Autodesk Inventor part; units mm, degrees
ref_plane "YZ Plane" through (0, 0, 0) normal (1, 0, 0) x (0, 1, 0)
ref_plane "XZ Plane" through (0, 0, 0) normal (0, 1, 0) x (-1, 0, 0)
ref_plane "XY Plane" through (0, 0, 0) normal (0, 0, 1) x (1, 0, 0)
sketch "Sketch1" plane through (0, 0, 0) normal (0, 0, 1) x (1, 0, 0)
  line L0 (0, 0) -> (25.4, 0)
  line L1 (25.4, 0) -> (25.4, 50.8)
  line L2 (25.4, 50.8) -> (0, 50.8)
  line L3 (0, 50.8) -> (0, 0)
  line L4 (23.8125, 1.5875) -> (1.5875, 1.5875)
  line L5 (1.5875, 1.5875) -> (1.5875, 49.2125)
  line L6 (1.5875, 49.2125) -> (23.8125, 49.2125)
  line L7 (23.8125, 49.2125) -> (23.8125, 1.5875)
  dimension "d0" = 25.4
  dimension "d1" = 50.8
  dimension "d2" = 1.5875
extrude "Extrusion1" add sketch "Sketch1" along normal blind 584.2
sketch "Sketch2" plane through (0, 50.8, 0) normal (0, 1, 0) x (1, 0, 0)
  line L0 (23.8125, 0) -> (1.5875, 0) construction
  line L1 (12.7, 0) -> (12.7, -12.7) construction
  line L2 (25.4, -584.2) -> (0, -584.2) construction
  line L3 (12.7, -584.2) -> (12.7, -571.5) construction
  circle A0 centre (12.7, -571.5) radius 2.5797
  circle A1 centre (12.7, -12.7) radius 2.5797
  point P0 (0, 0)
  dimension "d5" = 12.7
  dimension "d6" = 12.7
  dimension "d7" = 5.1594
extrude "Extrusion2" cut sketch "Sketch2" against normal blind 711.2
sketch "Sketch3" plane through (0, 50.8, 0) normal (0, 1, 0) x (1, 0, 0)
  circle A0 centre (12.7, -12.7) radius 2.5797 construction
  line L0 (12.7, -12.7) -> (12.7, -38.1) construction
  circle A1 centre (12.7, -38.1) radius 2.5797
  circle A2 centre (12.7, -571.5) radius 2.5797 construction
  line L1 (12.7, -571.5) -> (12.7, -546.1) construction
  circle A3 centre (12.7, -546.1) radius 2.5797
  point P0 (0, 0)
  dimension "d10" = 25.4
  dimension "d13" = 25.4
extrude "Extrusion4" cut sketch "Sketch3" against normal blind 68.2625
sketch "Sketch4" plane through (25.4, 0, 0) normal (1, 0, 0) x (0, 0, -1)
  line L0 (0, 0) -> (-584.2, 0) construction
  line L1 (0, 0) -> (-284.1625, 0) construction
  line L2 (-284.1625, 0) -> (-334.9625, 0) construction
  line L3 (-334.9625, 0) -> (-334.9625, 12.7) construction
  line L4 (-334.9625, 12.7) -> (-309.5625, 12.7) construction
  line L5 (-309.5625, 12.7) -> (-309.5625, 38.1) construction
  line L6 (-309.5625, 12.7) -> (-284.1625, 12.7) construction
  circle A0 centre (-284.1625, 12.7) radius 2.5797
  circle A1 centre (-334.9625, 12.7) radius 2.5797
  circle A2 centre (-309.5625, 38.1) radius 2.5797
  dimension "d16" = 284.1625
  dimension "d17" = 50.8
  dimension "d18" = 12.7
  dimension "d19" = 25.4
  dimension "d20" = 25.4
  dimension "d21" = 5.1594
  dimension "d22" = 5.1594
extrude "Extrusion5" cut sketch "Sketch4" against normal blind 25.4
sketch "Sketch5" plane through (0, 50.8, 0) normal (0, 1, 0) x (1, 0, 0)
  circle A0 centre (12.7, -38.1) radius 2.5797 construction
  line L0 (12.7, -38.1) -> (12.7, -63.5) construction
  circle A1 centre (12.7, -546.1) radius 2.5797 construction
  line L1 (12.7, -546.1) -> (12.7, -520.7) construction
  circle A2 centre (12.7, -520.7) radius 2.5797
  circle A3 centre (12.7, -63.5) radius 2.5797
  line L2 (12.7, -520.7) -> (12.7, -495.3) construction
  line L3 (12.7, -63.5) -> (12.7, -88.9) construction
  circle A4 centre (12.7, -88.9) radius 2.5797
  circle A5 centre (12.7, -495.3) radius 2.5797
  point P0 (0, 0)
  dimension "d25" = 25.4
  dimension "d26" = 25.4
  dimension "d29" = 25.4
  dimension "d30" = 25.4
extrude "Extrusion7" cut sketch "Sketch5" against normal blind 77.7875
properties part number "1x2 28in"
The listing builds one solid part. Answer for the finished solid, in the listing's coordinates (mm). A direction names the side the tool comes from. Coordinates: 2 decimals unless noted, no trailing zeros. Loops run counter-clockwise (first coordinate to the right, second up) from the corner with the lowest first, then second, coordinate; pieces in that order, holes last. Notation, with made-up numbers: (61, 49.25) -> (74, 49.25) arc R12 ccw to (74, 58.25) -> close; hole circle Ø3 at (57, 2). An arc over 180 degrees is marked (long way). Return JSON: item names as keys, results as strings. Group by question number.
(1) A cutting plane is placed at A-A on y = 30.5. Write down the section's boundary in (x, z).
(2) A cutting plane is placed at B-B on z = 267. Write down the section's boundary in (x, y).
(3) Find the intervals of material crossed by probe 1 along Y at (x, z) = (18.5, 64.5); probe 2 along X at (y, z) = (49.7, 88.9); probe 3 along X at (y, z) = (21.5, 288), in increasing order. Write a range as from..to.
(4) Determine the mould class of faces 3 (the flat face through (0, 26, 288)), 4 (the flat face through (1, 27, 0)), 5 (the flat face through (23.812, 26, 288)) for opening direction X: released by +X, released by -X, zero draft, split by the parting line, or undercut.
(5) Which of the six approach directions +Z, -Z, +X, -X, +Y, -Y give full straight-line access (tool end or side, diameter ignored) to faces 1 (the flat face through (13, 0, 288)), 2 (the flat face through (1.588, 25, 288))?
The answers:
{
 "1": {"outline": "(0, 0) -> (1.59, 0) -> (1.59, 584.2) -> (0, 584.2) -> close; (23.81, 0) -> (25.4, 0) -> (25.4, 584.2) -> (23.81, 584.2) -> close"},
 "2": {"outline": "(0, 0) -> (25.4, 0) -> (25.4, 50.8) -> (0, 50.8) -> close; hole (1.59, 1.59) -> (23.81, 1.59) -> (23.81, 49.21) -> (1.59, 49.21) -> close"},
 "3": {"probe 1": "y = 0..1.59, 49.21..50.8", "probe 2": "x = 0..10.12, 15.28..25.4", "probe 3": "x = 0..1.59, 23.81..25.4"},
 "4": {"face 3": "released by -X", "face 4": "zero draft", "face 5": "undercut"},
 "5": {"face 1": "+Z, -Z, +X, -X, -Y", "face 2": "+Z, -Z"}
}
